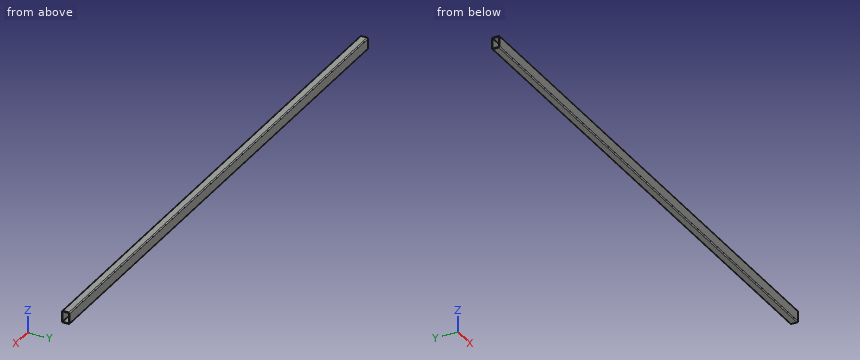
from build123d import *

# Parameters (mm, degrees)
F0_W     = 2867
F0_H     = 60
F1_DEPTH = 40
F2_T     = -3
F3_R     = 5
F4_R     = 1


with BuildPart() as f1:
    # F0 (on Front) → F1 (new body)
    with BuildSketch(Plane.XZ):
        with Locations((1433.5, 30)):
            Rectangle(F0_W, F0_H)
    extrude(amount=F1_DEPTH)

    # F2
    f2_openings = [f1.faces().sort_by_distance(p)[0] for p in [
        (0, -20, 30),
        (2867, -20, 30),
    ]]
    offset(amount=F2_T, openings=f2_openings)

    # F3
    f3_edges = [f1.edges().sort_by_distance(p)[0] for p in [
        (1433.5, -40, 60),
        (1433.5, -40, 0),
        (1433.5, 0, 0),
        (1433.5, 0, 60),
    ]]
    fillet(f3_edges, radius=F3_R)

    # F4
    f4_edges = [f1.edges().sort_by_distance(p)[0] for p in [
        (1433.5, -3, 3),
        (1433.5, -37, 3),
        (1433.5, -3, 57),
        (1433.5, -37, 57),
    ]]
    fillet(f4_edges, radius=F4_R)


solid = f1.part
Build history of the part. All positions in model axes, mm. Round coordinates to 2 decimals unless told otherwise and drop trailing zeros. Write each loop counter-clockwise with the first axis right and the second up, starting at its lowest first coordinate (ties: lowest second). Pieces come first, ordered by that corner, then holes. Notation, with made-up numbers: (-37.75, 36) -> (18.25, 36) arc R5 ccw to (18.25, 45) -> close; hole circle Ø10 at (-8, -14.5). An arc over 180 degrees is marked (long way). Write item = value, one per line.
(1) Band-saw the part on C-C (x = 1555.5). Give the cut face in (y, z).
Answer:
outline = (-40, 5) arc R5 ccw to (-35, 0) -> (-5, 0) arc R5 ccw to (0, 5) -> (0, 55) arc R5 ccw to (-5, 60) -> (-35, 60) arc R5 ccw to (-40, 55) -> close; hole (-37, 4) arc R1 ccw to (-36, 3) -> (-4, 3) arc R1 ccw to (-3, 4) -> (-3, 56) arc R1 ccw to (-4, 57) -> (-36, 57) arc R1 ccw to (-37, 56) -> close
(2) Band-saw the part on B-B (y = -23). Give the cut face in (x, z), then the cut area to 3 significant figures.
Answer:
outline = (0, 0) -> (2867, 0) -> (2867, 3) -> (0, 3) -> close; (0, 57) -> (2867, 57) -> (2867, 60) -> (0, 60) -> close
area = 17,200 mm2
(3) Probe L1, parallel to Y at x = 1794, z = 53.5; L2, parallel to Z at x = 2351.5, y = -16.5; L3, parallel to Y at x = 2531, z = 56.5. List the from-to ranges inside material, lowest first.
Answer:
L1 = -40 to -37, -3 to 0
L2 = 0 to 3, 57 to 60
L3 = -39.77 to -36.87, -3.13 to -0.23
(4) Band-saw the part on A-A (z = 42.5). Give the cut face in (x, y).
Answer:
outline = (0, -40) -> (2867, -40) -> (2867, -37) -> (0, -37) -> close; (0, -3) -> (2867, -3) -> (2867, 0) -> (0, 0) -> close
